Check sheet for the modelled part. Datum: model origin and axes. Units: mm. A direction names the side the tool comes from. Give positions to 0.01 mm unless a question says otherwise; leave off trailing zeros. Order: outer loops, then holes, each group sorted by start corner. A loop starts at its lowest first (then second) coordinate and runs counter-clockwise, first axis right, second up. Notation, with made-up numbers: (47, 87.25) -> (72, 87.25) arc R22 ccw to (72, 104.25) -> close; hole circle Ø11 at (0, 56). An arc over 180 degrees is marked (long way). One line per question, with ' | ' between items.
```python
from build123d import *

# Parameters (mm, degrees)
F0_W     = 250
F0_H     = 150
F7_DEPTH = 25
F1_R     = 7.5
F2_DEPTH = 35
F3_W     = 100
F3_H     = 100
F4_DEPTH = 100
F5_R     = 25
F8_DEPTH = 100.001
F6_R     = 49.99999


# Not quite as in the source:
# - a fillet or chamfer is up to 0.001 mm smaller than in the source, because OpenCascade refuses the exact size


with BuildPart() as f7:
    # F0 (on Top) → F7 (new body)
    with BuildSketch(Plane.XY):
        Rectangle(F0_W, F0_H)
    extrude(amount=F7_DEPTH)

    # F1 (on face) → F2 (join)
    with BuildSketch(Plane.XY.offset(25)):
        with Locations((-75, 0)):
            Circle(F1_R)
    extrude(amount=F2_DEPTH)

    # F3 (on face) → F4 (join)
    with BuildSketch(Plane.XY.offset(25)):
        with Locations((75, 0)):
            Rectangle(F3_W, F3_H)
    extrude(amount=F4_DEPTH)

    # F5 (on face) → F8 (cut, through all)
    with BuildSketch(Plane(origin=(25, 0, 0), x_dir=(0, -1, 0), z_dir=(-1, 0, 0))):
        with Locations((0, 75)):
            Circle(F5_R)
    extrude(amount=-F8_DEPTH, mode=Mode.SUBTRACT)

    # F6 (radius 50 in the source; OpenCascade refuses exactly that, so slightly less here)
    f6_edges = [f7.edges().sort_by_distance(p)[0] for p in [
        (75, 50, 125),
        (75, -50, 125),
    ]]
    fillet(f6_edges, radius=F6_R)


solid = f7.part
```
Q1. Section check C-C (y = 34.5). Enter the section's corners in (x, z), and give its area (3 significant figures).
Result sheet:
outline: (-125, 0) -> (125, 0) -> (125, 111.19) -> (25, 111.19) -> (25, 25) -> (-125, 25) -> close | area: 14,900 mm2
Q2. Access from +Z, -Z, +X, -X, +Y, -Y to the whole of each face (thin tool, end or side, straight path). Record for faces 1 (the face through (74, -50, 50)), 2 (the face through (74, 50, 50)), 3 (the face through (125, -1, 48)).
Result sheet:
face 1: +Z, +X, -X, -Y | face 2: +Z, +X, -X, +Y | face 3: +Z, -Z, +X, +Y, -Y
Q3. Section check D-D (x = 14). Enter the section's corners in (y, z), and give its area (3 significant figures).
Result sheet:
outline: (-75, 0) -> (75, 0) -> (75, 25) -> (-75, 25) -> close | area: 3,750 mm2
Q4. Depth check by flat-ended pin: pin 1 Ø10 at (x, y) = (-28.5, -9) entering from +Z; pin 2 Ø7.5 at (x, y) = (-75, -2) entering from +Z; pin 3 Ø12 at (x, z) = (-84, 54.5) entering from +Y. Enter the tip coordinate at first touch or a pass-through.
Result sheet:
pin 1: stops at z = 25 | pin 2: stops at z = 60 | pin 3: stops at y = 6.87
Q5. Section check B-B (x = -75). Enter the section's corners in (y, z), and give its area (4 significant figures).
Result sheet:
outline: (-75, 0) -> (75, 0) -> (75, 25) -> (7.5, 25) -> (7.5, 60) -> (-7.5, 60) -> (-7.5, 25) -> (-75, 25) -> close | area: 4,275 mm2
Q6. Thickness scan on line 1 (Y direction, x = 65, z = 73.5); line 2 (X direction, y = -11, z = 49); line 3 (Z direction, x = -33, y = -39). Record the ranges inside material, lowest first.
Result sheet:
line 1: y = -50 to -24.95, 24.95 to 50 | line 2: x = 25 to 125 | line 3: z = 0 to 25
Q7. Mould release check, pull along X, two halves, no side actions. Record for faces 4 (the face through (-82.493, 0.33, 42.255)), 5 (the face through (-125, -1, 12)), 6 (the face through (-2, 1, 0)): pulls with the +X half, pulls with the -X half, needs draft (parallel to the pull), parting line crosses it, or undercut.
Result sheet:
face 4: undercut | face 5: pulls with the -X half | face 6: needs draft
